Design review of the part shown in the three views and the two pictorial views. Dimensions are in mm from the part's minimum x, y and z. A direction names the side the tool comes from. Give positions to 0.01 mm unless a question says otherwise; leave off trailing zeros. Order: outer loops, then holes, each group sorted by start corner. A loop starts at its lowest first (then second) coordinate and runs counter-clockwise, first axis right, second up.
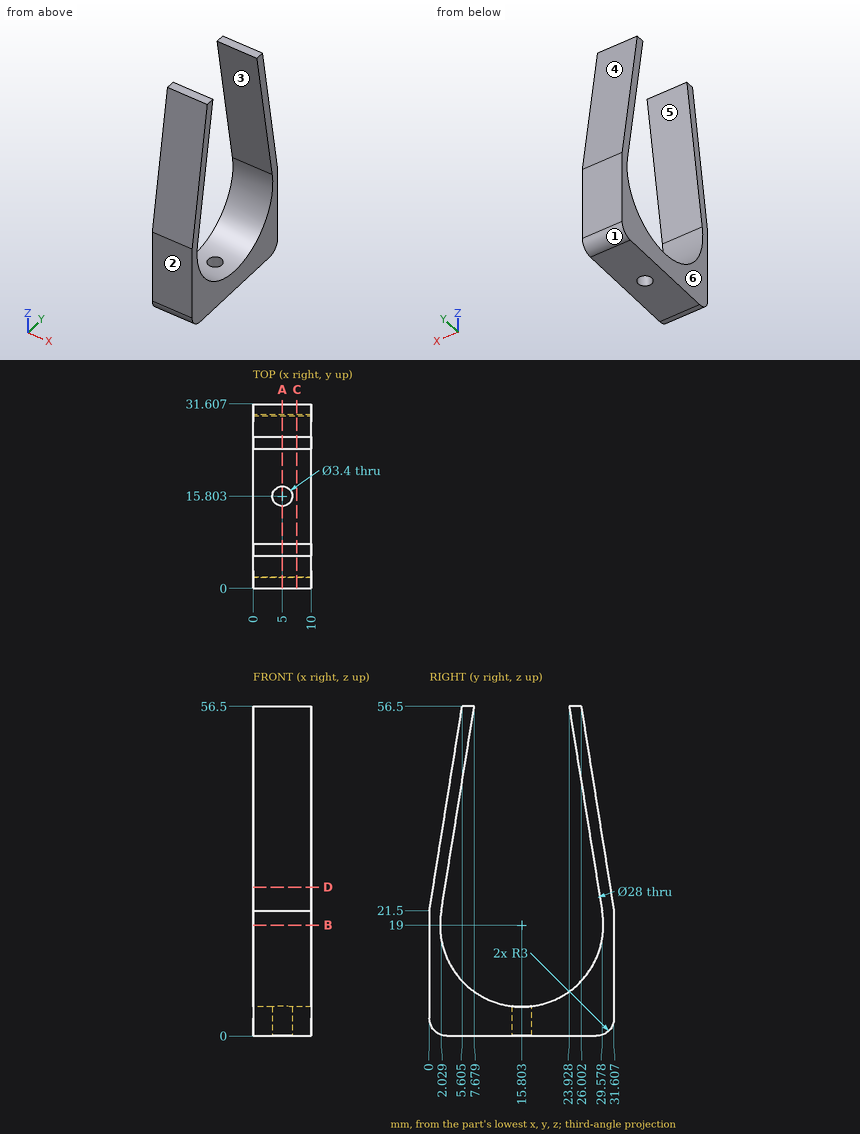
1) Clearance check with flat-ended pins moving along their axes: pin 1 (2 mm diameter, centred on x = 5, y = 15.8, fed in from -Z); pin 2 (4 mm diameter, centred on x = 3.5, z = 37, fed in from +Y) (1 decimal); pin 3 (6 mm diameter, centred on x = 4.5, y = 19.5, fed in from +Z) (1 decimal). State where each tip first meets the part, or that it passes through.
Answer sheet:
pin 1: passes through
pin 2: stops at y = 29.4
pin 3: stops at z = 6.7
2) To check wall thickness, follow line 1 (Y direction, x = 6.75, z = 24) (1 decimal); line 2 (Y direction, x = 8, z = 20.5) (1 decimal); line 3 (Z direction, x = 8.5, y = 14). State the ranges of each line that lie inside material, in increasing order.
Answer sheet:
line 1: y = 0.4 to 2.4, 29.2 to 31.2
line 2: y = 0 to 1.9, 29.7 to 31.6
line 3: z = 0 to 5.12
3) Tool access review of the marked faces 5 and 6: name each direction out of +Z, -Z, +X, -X, +Y, -Y from which nothing blocks a thin tool from reaching the whole face with its end or side.
Answer sheet:
face 5: +X, -X
face 6: +Z, -Z, -X, +Y, -Y
4) We need section C-C on x = 7.5. Give the boundary of the cut face in (y, z) (1 decimal), then the cut area to 3 significant figures.
Answer sheet:
outline: (0, 3) arc R3 ccw to (3, 0) - (28.6, 0) arc R3 ccw to (31.6, 3) - (31.6, 21.5) - (26, 56.5) - (23.9, 56.5) - (29.6, 21.5) arc R14 cw (long way) to (2, 21.5) - (7.7, 56.5) - (5.6, 56.5) - (0, 21.5) - close
area: 442 mm2
5) We need section A-A on x = 5. Give the boundary of the cut face in (y, z) (1 decimal).
Answer sheet:
outline: (0, 3) arc R3 ccw to (3, 0) - (14.1, 0) - (14.1, 5.1) arc R14 cw to (2, 21.5) - (7.7, 56.5) - (5.6, 56.5) - (0, 21.5) - close; (17.5, 0) - (28.6, 0) arc R3 ccw to (31.6, 3) - (31.6, 21.5) - (26, 56.5) - (23.9, 56.5) - (29.6, 21.5) arc R14 cw to (17.5, 5.1) - close
6) We need section B-B on z = 19. Give the boundary of the cut face in (x, y).
Answer sheet:
outline: (0, 0) - (10, 0) - (10, 1.8) - (0, 1.8) - close; (0, 29.8) - (10, 29.8) - (10, 31.61) - (0, 31.61) - close
7) We need section D-D on z = 25.5. Give the boundary of the cut face in (x, y) (1 decimal).
Answer sheet:
outline: (0, 0.6) - (10, 0.6) - (10, 2.7) - (0, 2.7) - close; (0, 28.9) - (10, 28.9) - (10, 31) - (0, 31) - close
8) Draft analysis for pull direction Z (two halves, no side actions). For the marked faces 1, 2, 3 and 4, state which applies: +Z half, -Z half, draft (parallel to the pull), parting line (faces both ways), or undercut.
Answer sheet:
face 1: -Z half
face 2: draft
face 3: undercut
face 4: +Z half
